Could you check a few things on this model? Use its own coordinates, in mm. A direction names the side the tool comes from. Round coordinates to 2 decimals unless told otherwise and drop trailing zeros. Loops run counter-clockwise (first coordinate to the right, second up) from the corner with the lowest first, then second, coordinate; pieces in that order, holes last. Notation, with made-up numbers: (14, 18) -> (18, 18) arc R16 cw to (18, 26) -> close; hole circle Ø4 at (-36.75, 4.5). An arc over 180 degrees is marked (long way). Put each result on its own line as item: value. Start each with the question number.
1. Imagine slicing it at A-A, the plane y = 20. Please give me the cut outline in (x, z) (3 decimals).
2. Imagine slicing it at C-C, the plane x = 17.5. Please give me the cut outline in (y, z) (3 decimals), and give its area (3 significant figures).
3. Which directions (+Z, -Z, +X, -X, +Y, -Y) give clear straight access to the entire face, cutting with the end or side of a thin tool? Please do faces 1 (the flat face through (20.203, 61, 2)), 2 (the flat face through (0, 39, 2)).
4. If we mould it in two halves opening along X, with no side actions, what happens to faces 3 (the flat face through (50.203, 39, 2)), 4 (the flat face through (7, 13.648, 2)), 5 (the cylindrical face through (13.331, 27.097, 1.565)), 6 (the cylindrical face through (24.835, 25.874, 1.565))? For each: pulls with the +X half, pulls with the -X half, needs draft (parallel to the pull), parting line crosses it, or undercut.
5. Imagine slicing it at D-D, the plane x = 33.5. Please give me the cut outline in (y, z) (3 decimals), and give its area (3 significant figures).
6. Imagine slicing it at B-B, the plane z = 2.4. Please give me the cut outline in (x, y).
7. I'm going to push a flat-ended pin straight in: P1, Ø1, axis at y = 61.5, z = 2.5, coming from the -X side. Where does the tip first touch, or does it pass through?
8. I need wall thicknesses on line 1 (X direction, y = 25, z = 1.7); line 2 (Y direction, x = 25.5, z = 0.6); line 3 (X direction, y = 21, z = 0.7). Which ranges of each line are inside material? Lowest first, please. Write a range as [from, to].
Autodesk Inventor part; units mm, degrees
ref_plane "YZ Plane" through (0, 0, 0) normal (1, 0, 0) x (0, 1, 0)
ref_plane "XZ Plane" through (0, 0, 0) normal (0, 1, 0) x (-1, 0, 0)
ref_plane "XY Plane" through (0, 0, 0) normal (0, 0, 1) x (1, 0, 0)
sketch "Sketch1" plane through (0, 0, 0) normal (0, 0, 1) x (1, 0, 0)
  line L0 (20.2032, 59.7234) -> (20.2032, 63)
  line L1 (20.2032, 63) -> (0, 63)
  line L2 (0, 63) -> (0, 60)
  line L3 (30, 59.7234) -> (30, 63)
  line L4 (30, 63) -> (50.2032, 63)
  line L5 (50.2032, 63) -> (50.2032, 60)
  line L6 (30, 59.7234) -> (20.2032, 59.7234)
  circle A0 centre (13.6016, 25.8766) radius 1.25
  circle A1 centre (36.5, 25.6) radius 1.25
  line L7 (20.2032, 59.7234) -> (20.2032, 63)
  line L8 (20.2032, 63) -> (0, 63)
  line L9 (0, 63) -> (0, 60)
  line L10 (30, 59.7234) -> (30, 63)
  line L11 (30, 63) -> (50.2032, 63)
  line L12 (50.2032, 63) -> (50.2032, 60)
  line L13 (30, 59.7234) -> (20.2032, 59.7234)
  circle A2 centre (13.6016, 25.8766) radius 1.25
  circle A3 centre (36.5, 25.6) radius 1.25
  line L14 (0, 60) -> (0, 13.648)
  line L15 (50.2032, 60) -> (50.2032, 13.648)
  line L16 (0, 13.648) -> (13.2196, 13.648)
  line L17 (50.2032, 13.648) -> (36.9836, 13.648)
  arc A4 (36.9836, 13.648) -> (13.2196, 13.648) centre (25.1016, 13.9897) ccw
  point P0 (0, 0)
  dimension "d0" = 20.2032
  dimension "d1" = 3.2766
  dimension "d2" = 20.2032
  dimension "d3" = 2.5
  dimension "d4" = 2.5
  dimension "d7" = 20.2032
  dimension "d8" = 3.2766
  dimension "d9" = 20.2032
  dimension "d10" = 2.5
  dimension "d11" = 2.5
  dimension "d14" = 46.352
  dimension "d15" = 13.2196
  dimension "d16" = 13.2196
extrude "Extrusion1" add sketch "Sketch1" along normal blind 3.175
equation "\"d0\" = d5"
equation "\"d1\" = d6"
equation "\"d2\" = d5"
equation "\"d7\" = d12"
equation "\"d8\" = d13"
equation "\"d9\" = d12"
equation "\"d16\" = d15"
properties part number "side_plate_top"
Entries:
1. outline: (0, 0) -> (14.846, 0) -> (14.846, 3.175) -> (0, 3.175) -> close; (35.357, 0) -> (50.203, 0) -> (50.203, 3.175) -> (35.357, 3.175) -> close
2. outline: (23.128, 0) -> (63, 0) -> (63, 3.175) -> (23.128, 3.175) -> close
2. area: 127 mm^2
3. face 1: +Z, -Z, +Y
3. face 2: +Z, -Z, -X, +Y, -Y
4. face 3: pulls with the +X half
4. face 4: needs draft
4. face 5: undercut
4. face 6: undercut
5. outline: (22.402, 0) -> (63, 0) -> (63, 3.175) -> (22.402, 3.175) -> close
5. area: 129 mm^2
6. outline: (0, 13.65) -> (13.22, 13.65) arc R11.89 cw (long way) to (36.98, 13.65) -> (50.2, 13.65) -> (50.2, 63) -> (30, 63) -> (30, 59.72) -> (20.2, 59.72) -> (20.2, 63) -> (0, 63) -> close; hole circle Ø2.5 at (13.6, 25.88); hole circle Ø2.5 at (36.5, 25.6)
7. P1: x = 0
8. line 1: [0, 12.71], [14.49, 20.62], [29.58, 35.4], [37.6, 50.2]
8. line 2: [25.87, 59.72]
8. line 3: [0, 15.5], [34.7, 50.2]
